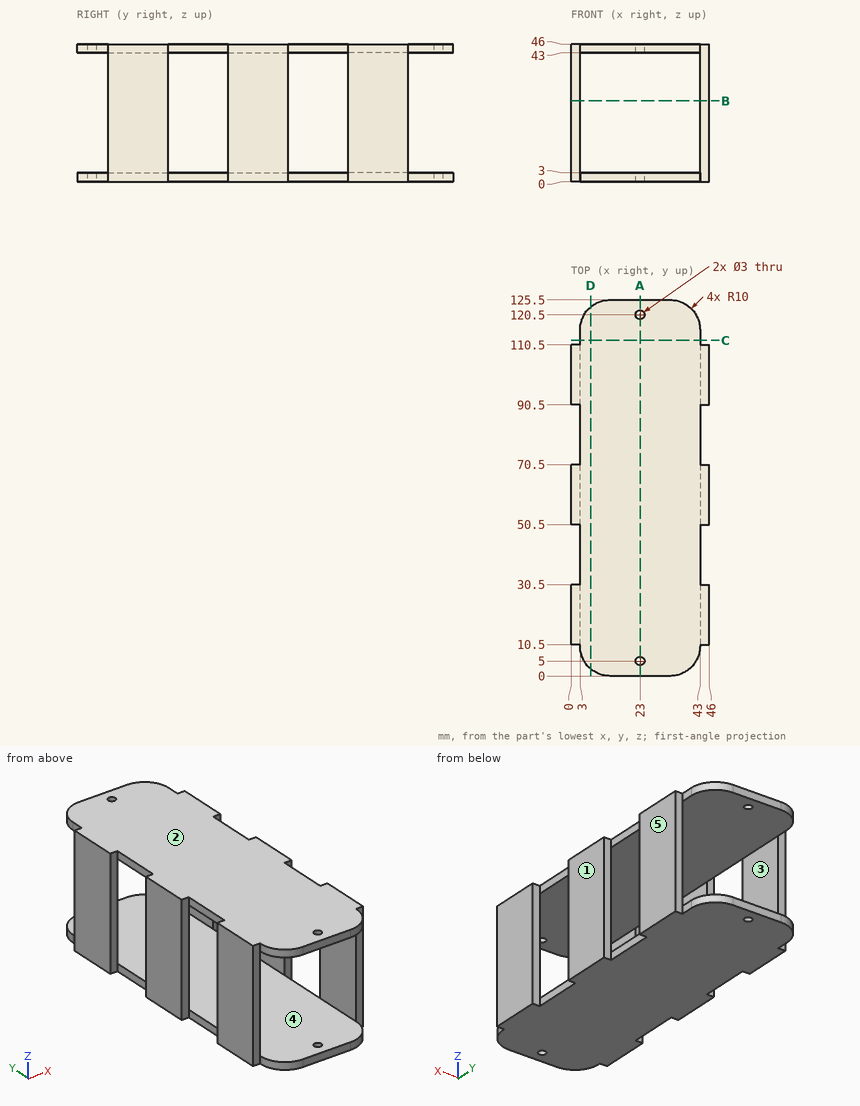
Geometry: see drawing. Coordinates: mm, zero at the bounding-box minimum. A direction names the side the tool comes from. Give positions to 0.01 mm unless a question says otherwise; leave off trailing zeros. Order: outer loops, then holes, each group sorted by start corner. A loop starts at its lowest first (then second) coordinate and runs counter-clockwise, first axis right, second up. Notation, with made-up numbers: (74, 7) - (109, 7) arc R20 ccw to (109, 37) - close; hole circle Ø1 at (-9.75, -36). An arc over 180 degrees is marked (long way). Use a Markdown table: item, result.
(1) Section query D-D (x = 6.5). Output: boundary loops of the cut face in (y, z).
Computed values:
| item | result |
|---|---|
| outline | (2.4, 0) - (123.1, 0) - (123.1, 3) - (2.4, 3) - close; (2.4, 43) - (123.1, 43) - (123.1, 46) - (2.4, 46) - close |
(2) Section query A-A (x = 23). Output: boundary loops of the cut face in (y, z).
Computed values:
| item | result |
|---|---|
| outline | (0, 0) - (3.5, 0) - (3.5, 3) - (0, 3) - close; (0, 43) - (3.5, 43) - (3.5, 46) - (0, 46) - close; (6.5, 0) - (119, 0) - (119, 3) - (6.5, 3) - close; (6.5, 43) - (119, 43) - (119, 46) - (6.5, 46) - close; (122, 0) - (125.5, 0) - (125.5, 3) - (122, 3) - close; (122, 43) - (125.5, 43) - (125.5, 46) - (122, 46) - close |
(3) Line query: line 1 (Y direction, x = 23, z = 44.8); line 2 (Z direction, x = 41, y = 46). Output: solid intervals per line, ascending. Write a range as from..to.
Computed values:
| item | result |
|---|---|
| line 1 | y = 0..3.5, 6.5..119, 122..125.5 |
| line 2 | z = 0..3, 43..46 |
(4) Section query C-C (y = 112). Output: boundary loops of the cut face in (x, z), then the cut area to 3 significant figures.
Computed values:
| item | result |
|---|---|
| outline | (3, 0) - (43, 0) - (43, 3) - (3, 3) - close; (3, 43) - (43, 43) - (43, 46) - (3, 46) - close |
| area | 240 mm2 |
(5) Access query for the marked faces 4 and 5. Directions: +Z, -Z, +X, -X, +Y, -Y. A direction counts if a zero-diameter tool reaches every point of the face in a straight line with its end or side. Return the directions, or none.
Computed values:
| item | result |
|---|---|
| face 4 | +Y, -Y |
| face 5 | +Z, -Z, +X, +Y, -Y |
(6) Section query B-B (z = 27). Output: boundary loops of the cut face in (x, y).
Computed values:
| item | result |
|---|---|
| outline | (0, 10.5) - (3, 10.5) - (3, 30.5) - (0, 30.5) - close; (0, 50.5) - (3, 50.5) - (3, 70.5) - (0, 70.5) - close; (0, 90.5) - (3, 90.5) - (3, 110.5) - (0, 110.5) - close; (43, 10.5) - (46, 10.5) - (46, 30.5) - (43, 30.5) - close; (43, 50.5) - (46, 50.5) - (46, 70.5) - (43, 70.5) - close; (43, 90.5) - (46, 90.5) - (46, 110.5) - (43, 110.5) - close |
(7) Pin query (flat end, axial travel): pin 1 (1.5 mm diameter, centred on x = 2, z = 31.5, fed in from +Y); pin 2 (3.5 mm diameter, centred on y = 78, z = 1, fed in from -X); pin 3 (0.9 mm diameter, centred on x = 1.5, z = 31, fed in from -Y). Return the tip coordinate at first contact, or that it passes through.
Computed values:
| item | result |
|---|---|
| pin 1 | stops at y = 110.5 |
| pin 2 | stops at x = 3 |
| pin 3 | stops at y = 10.5 |
(8) Draft query along Z for the marked faces 1, 2 and 3. Return one class per face: released by +Z, released by -Z, zero draft, split by the parting line, or undercut.
Computed values:
| item | result |
|---|---|
| face 1 | zero draft |
| face 2 | released by +Z |
| face 3 | undercut |
